```python
from build123d import *

# Parameters (mm, degrees)
SKETCH1_W                      = 30
SKETCH1_H                      = 26
BOSS_EXTRUDE1_DEPTH            = 25
CUT_EXTRUDE3_DEPTH             = 3.5
F_3_7_3_7_DIAMETER_HOLE1_D     = 3.7
F_3_7_3_7_DIAMETER_HOLE1_DEPTH = 4
F_3_7_3_7_DIAMETER_HOLE1_TIP   = 1.111592145
F_2_7_2_7_DIAMETER_HOLE3_D     = 2.7
F_2_7_2_7_DIAMETER_HOLE3_DEPTH = 12
F_2_7_2_7_DIAMETER_HOLE3_TIP   = 0.811161836
FILLET1_R                      = 6
CHAMFER1_SIZE                  = 0.5


with BuildPart() as part:
    # Sketch1 → Boss-Extrude1 (new body)
    with BuildSketch(Plane(origin=(0, 0, 0), x_dir=(1, 0, 0), z_dir=(0, 1, 0))):
        Rectangle(SKETCH1_W, SKETCH1_H)
    extrude(amount=BOSS_EXTRUDE1_DEPTH)

    # Sketch12 → Cut-Extrude3 (cut)
    with BuildSketch(Plane.XZ):
        with BuildLine():
            Line((13.059862174, 6.3), (-13.059862174, 6.3))
            ThreePointArc((-13.059862174, 6.3), (-14.5, 0), (-13.059862174, -6.3))
            Line((-13.059862174, -6.3), (13.059862174, -6.3))
            ThreePointArc((13.059862174, -6.3), (14.5, 0), (13.059862174, 6.3))
        make_face()
    extrude(amount=-CUT_EXTRUDE3_DEPTH, mode=Mode.SUBTRACT)

    # Ø3.7 (3.7) Diameter Hole1
    with Locations(Plane.XY.offset(13)):
        with Locations((7, 5.5), (7, 19.5), (-7, 5.5), (-7, 19.5)):
            Hole(F_3_7_3_7_DIAMETER_HOLE1_D / 2, depth=F_3_7_3_7_DIAMETER_HOLE1_DEPTH)
            with Locations((0, 0, -(F_3_7_3_7_DIAMETER_HOLE1_DEPTH + F_3_7_3_7_DIAMETER_HOLE1_TIP / 2))):  # 118° drill point
                Cone(0, F_3_7_3_7_DIAMETER_HOLE1_D / 2, F_3_7_3_7_DIAMETER_HOLE1_TIP, mode=Mode.SUBTRACT)

    # Sketch13 → Cut-Revolve2 (revolve, cut)
    with BuildSketch(Plane.XY, mode=Mode.PRIVATE) as cut_revolve2_sk:
        Polygon((-6.6, 0), (-6.6, 23.1), (-4.75, 23.1), (-4.75, 25), (0, 25), (0, 0), align=None)
    revolve(cut_revolve2_sk.sketch.rotate(Axis((0, 0, 0), (0, 1, 0)), 270), axis=Axis((0, 0, 0), (0, 1, 0)), mode=Mode.SUBTRACT)

    # Ø2.7 (2.7) Diameter Hole3
    with Locations(Plane.XZ.offset(-3.5)):
        with Locations((-9.25, 0), (9.25, 0)):
            Hole(F_2_7_2_7_DIAMETER_HOLE3_D / 2, depth=F_2_7_2_7_DIAMETER_HOLE3_DEPTH)
            with Locations((0, 0, -(F_2_7_2_7_DIAMETER_HOLE3_DEPTH + F_2_7_2_7_DIAMETER_HOLE3_TIP / 2))):  # 118° drill point
                Cone(0, F_2_7_2_7_DIAMETER_HOLE3_D / 2, F_2_7_2_7_DIAMETER_HOLE3_TIP, mode=Mode.SUBTRACT)

    # Fillet1
    fillet1_edges = [part.edges().sort_by_distance(p)[0] for p in [
        (-15, 12.5, -13),
        (15, 12.5, -13),
    ]]
    fillet(fillet1_edges, radius=FILLET1_R)

    # Chamfer1
    chamfer1_edges = [part.edges().sort_by_distance(p)[0] for p in [
        (15, 25, 3),
        (0, 25, 4.75),
        (0, 25, -13),
        (-15, 25, 3),
        (-13.242640687, 25, -11.242640687),
        (13.242640687, 25, -11.242640687),
        (0, 25, 13),
    ]]
    chamfer(chamfer1_edges, length=CHAMFER1_SIZE)


solid = part.part
```
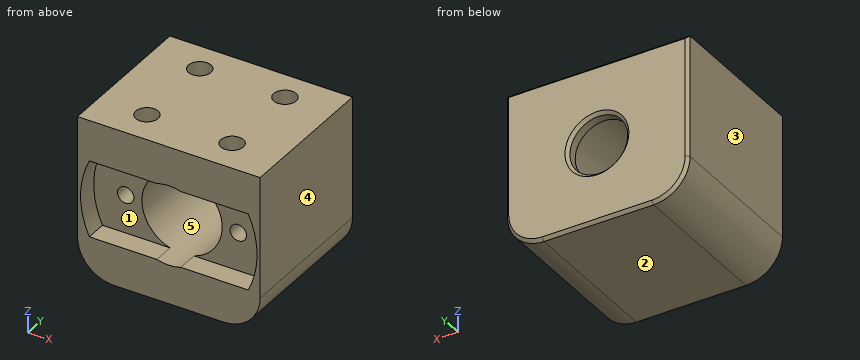
Source: CAD feature listing. Evaluate the final solid. Frame: model axes, mm. Face numbers are marked on the shaded views. A direction names the side the tool comes from. Give positions to 0.01 mm unless a question says otherwise; leave off trailing zeros. Loops run counter-clockwise (first coordinate to the right, second up) from the corner with the lowest first, then second, coordinate; pieces in that order, holes last. Notation, with made-up numbers: (62.5, -5) -> (108.5, -5) arc R16 cw to (108.5, 16) -> close; hole circle Ø10 at (53.5, -4.5). An arc over 180 degrees is marked (long way). Put each result on its own line as item: value. Start each with the question number.
1) Draft query along Z for the marked faces 1, 2 and 3. Return one class per face: released by +Z, released by -Z, zero draft, split by the parting line, or undercut.
2) Cut plane A-A (x = 0). Return loops of the section in (y, z), then the cut area to 3 significant figures.
3) Cut plane C-C (y = 6.75). State how many separate pieces and enclosed holes the cut face has, then the cut area to 3 significant figures.
4) Contact query for flat-ended pins moving along their axis: P1, Ø10, axis at x = 5.5, z = -1, coming from the -Y side; P2, Ø2, axis at x = -7, y = 5.5, coming from the +Z side; P3, Ø1.6, axis at x = 9.25, z = 0, coming from the -Y side. Output: stop coordinate, or through.
5) Material intervals for probe 1 along X at (y, z) = (8, 0); probe 2 along X at (y, z) = (5.5, 11.6); probe 3 along X at (y, z) = (16.75, 0), sorted ascending.
6) Cut plane B-B (z = 10.5). Return loops of the section in (x, y), then the cut area to 3 significant figures.
7) Reachability of the marked faces 4 and 5 from +Z, -Z, +X, -X, +Y, -Y: full face, straight path, thin tool, end or side. Return the list, or none.
Results are:
1. face 1: undercut
1. face 2: released by -Z
1. face 3: zero draft
2. outline: (0, -13) -> (24.5, -13) -> (25, -12.5) -> (25, -5.25) -> (24.5, -4.75) -> (23.1, -4.75) -> (23.1, -6.6) -> (0, -6.6) -> close; (0, 6.6) -> (23.1, 6.6) -> (23.1, 4.75) -> (24.5, 4.75) -> (25, 5.25) -> (25, 12.5) -> (24.5, 13) -> (0, 13) -> close
2. area: 327 mm2
3. separate pieces: 1
3. enclosed holes: 3
3. area: 593 mm2
4. P1: stops at y = 3.5
4. P2: stops at z = 8.49
4. P3: stops at y = 15.83
5. probe 1: x = -15 to -10.6, -7.9 to -6.6, 6.6 to 7.9, 10.6 to 15
5. probe 2: x = -15 to -8.85, -5.15 to 5.15, 8.85 to 15
5. probe 3: x = -15 to -6.6, 6.6 to 15
6. outline: (-15, 0) -> (15, 0) -> (15, 24.5) -> (14.5, 25) -> (-14.5, 25) -> (-15, 24.5) -> close; hole circle Ø3.7 at (-7, 5.5); hole circle Ø3.7 at (-7, 19.5); hole circle Ø3.7 at (7, 5.5); hole circle Ø3.7 at (7, 19.5)
6. area: 707 mm2
7. face 4: +Z, -Z, +X, +Y, -Y
7. face 5: -Y
